```python
from build123d import *

# Parameters (mm, degrees)
BOX133_W           = 3.5
BOX133_H           = 31
BOX133_DEPTH       = 4
CHAMFER022_1_SIZE2 = 14
CHAMFER022_1_SIZE  = 3.9
CHAMFER022_2_SIZE2 = 14
CHAMFER022_2_SIZE  = 3.9


with BuildPart() as part:
    # Box133 → Box133 (new body)
    with BuildSketch(Plane(origin=(26, -16.5, 6), x_dir=(1, 0, 0), z_dir=(0, 0, 1))):
        with Locations((1.75, 15.5)):
            Rectangle(BOX133_W, BOX133_H)
    extrude(amount=BOX133_DEPTH)

    # Chamfer022 1
    chamfer022_1_edges = [part.edges().sort_by_distance(p)[0] for p in [
        (27.75, 14.5, 6),
    ]]
    chamfer022_1_side = part.faces().sort_by_distance((27.75, 14.5, 8))[0]
    chamfer(chamfer022_1_edges, length=CHAMFER022_1_SIZE, length2=CHAMFER022_1_SIZE2, reference=chamfer022_1_side)

    # Chamfer022 2
    chamfer022_2_edges = [part.edges().sort_by_distance(p)[0] for p in [
        (27.75, -16.5, 6),
    ]]
    chamfer022_2_side = part.faces().sort_by_distance((27.75, -16.5, 8))[0]
    chamfer(chamfer022_2_edges, length=CHAMFER022_2_SIZE, length2=CHAMFER022_2_SIZE2, reference=chamfer022_2_side)


with BuildPart() as part_1:
    # Chamfer022 placement: moved
    add(part.part.moved(Location((0, 1, -1))))


solid = part_1.part
```
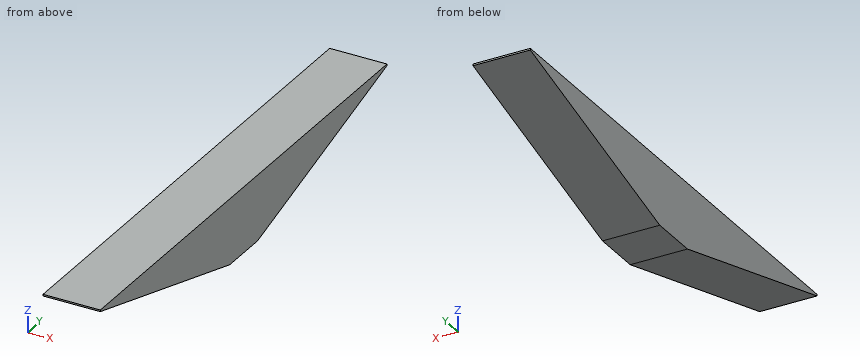
Source: CAD feature listing. Evaluate the final solid. Frame: model axes, mm. Round coordinates to 2 decimals unless told otherwise and drop trailing zeros. Loops run counter-clockwise (first coordinate to the right, second up) from the corner with the lowest first, then second, coordinate; pieces in that order, holes last. Notation, with made-up numbers: (-32.75, 65.25) - (-5.75, 65.25) arc R13 ccw to (-5.75, 76.25) - close; hole circle Ø4 at (36, 57). An arc over 180 degrees is marked (long way). Use CSV: the item, a comma, the result in double quotes.
Q1. Section query C-C, the plane z = 5.45. Output: boundary loops of the cut face in (x, y), then the cut area to 3 significant figures.
Reported:
outline,"(26, -3.12) - (29.5, -3.12) - (29.5, 3.12) - (26, 3.12) - close"
area,"21.8 mm^2"
Q2. Section query A-A, the plane x = 28.25. Output: boundary loops of the cut face in (y, z), then the cut area to 3 significant figures.
Reported:
outline,"(-15.5, 8.9) - (-1.5, 5) - (1.5, 5) - (15.5, 8.9) - (15.5, 9) - (-15.5, 9) - close"
area,"69.4 mm^2"
Q3. Ray query, line 1 along Z through (x, y) = (27.45, 11); line 2 along Z through (x, y) = (26.8, -8). Return the intervals inside material, ascending.
Reported:
line 1,"7.65 to 9"
line 2,"6.81 to 9"
Q4. Section query B-B, the plane y = 8.5. Output: boundary loops of the cut face in (x, z), then the cut area to 4 significant figures.
Reported:
outline,"(26, 6.95) - (29.5, 6.95) - (29.5, 9) - (26, 9) - close"
area,"7.175 mm^2"
